Geometry: final body of the model. Coordinates: model frame, mm. A direction names the side the tool comes from. Give positions to 0.01 mm unless a question says otherwise; leave off trailing zeros. Write each loop counter-clockwise with the first axis right and the second up, starting at its lowest first coordinate (ties: lowest second). Pieces come first, ordered by that corner, then holes. Notation, with made-up numbers: (57.25, -22.5) -> (97.25, -22.5) arc R21 cw to (97.25, 16.5) -> close; hole circle Ø8 at (21.5, 42). An arc over 180 degrees is marked (long way). Use CSV: the item, a comma, the result in double quotes. Start each with the question number.
1) Set-up query: faces 1 (the face through (0, 12, 1)), 2 (the face through (0, 5, 2.5)). Return all of +Z, -Z, +X, -X, +Y, -Y with unobstructed straight access to the full face (end or side cutting, diameter ignored); none if empty.
2) Section B-B (x = 0). Output: boundary loops of the cut face in (y, z), plus the area to 3 significant figures.
3) Contact query for flat-ended pins moving along their axis: P1, Ø2, axis at y = -9.5, z = 3.5, coming from the -X side; P2, Ø1.5, axis at x = -2, z = 2.5, coming from the -Y side; P3, Ø2, axis at y = -15, z = 1.5, coming from the +X side; P4, Ø5, axis at x = 0, y = 0, coming from the +Z side. Output: stop coordinate, or through.
4) Material intervals for line 1 (X direction, y = 0, z = 0.8); line 2 (X direction, y = 0, z = 2.05); line 3 (Z direction, x = 1.5, y = 9), sorted ascending. Write a range as [from, to].
5) Section C-C (z = 0.6). Output: boundary loops of the cut face in (x, y).
6) Draft query along Y for faces 3 (the face through (1, -16, 4)), 4 (the face through (0.148, -6.157, 2.533)), 5 (the face through (-10, 0, 1)). Return one class per face: pulls with the +Y half, pulls with the -Y half, needs draft (parallel to the pull), parting line crosses it, or undercut.
7) Section D-D (y = -15). Output: boundary loops of the cut face in (x, z), plus the area to 3 significant figures.
8) Section A-A (y = 0). Output: boundary loops of the cut face in (x, z).
```python
from build123d import *

# Parameters (mm, degrees)
ESQUISSE1_R             = 4
ESQUISSE1_R_2           = 1.2
ESQUISSE1_R_3           = 1.5
BOSS_EXTRU_1_DEPTH      = 4
ENL_V_MAT_EXTRU_1_DEPTH = 25
CHANFREIN1_SIZE         = 1
CONG_1_R                = 4


with BuildPart() as part:
    # Esquisse1 → Boss.-Extru.1 (new body)
    with BuildSketch(Plane.XY):
        with BuildLine():
            Line((-10.150862032, -6.4), (-3.383620677, -17.133333333))
            ThreePointArc((-3.383620677, -17.133333333), (0, -19), (3.383620677, -17.133333333))
            Line((3.383620677, -17.133333333), (10.150862032, -6.4))
            ThreePointArc((10.150862032, -6.4), (0, 12), (-10.150862032, -6.4))
        make_face()
        Circle(ESQUISSE1_R, mode=Mode.SUBTRACT)
        with Locations((0, -15)):
            Circle(ESQUISSE1_R_2, mode=Mode.SUBTRACT)
        with Locations((-8.5, 0)):
            Circle(ESQUISSE1_R_3, mode=Mode.SUBTRACT)
        with Locations((8.5, 0)):
            Circle(ESQUISSE1_R_3, mode=Mode.SUBTRACT)
    extrude(amount=BOSS_EXTRU_1_DEPTH)

    # Esquisse2 → Enlèv. mat.-Extru.1 (cut, symmetric)
    with BuildSketch(Plane(origin=(0, 0, 0), x_dir=(0, 0, -1), z_dir=(1, 0, 0))):
        Polygon((-4, -11.766666667), (-2.5, -6.168590455), (-2.5, 12), (-4, 12), align=None)
    extrude(amount=ENL_V_MAT_EXTRU_1_DEPTH, both=True, mode=Mode.SUBTRACT)

    # Chanfrein1
    chanfrein1_edges = [part.edges().sort_by_distance(p)[0] for p in [
        (-10, 0, 2.5),
        (7, 0, 2.5),
    ]]
    chamfer(chanfrein1_edges, length=CHANFREIN1_SIZE)

    # Congé1
    cong_1_edges = [part.edges().sort_by_distance(p)[0] for p in [
        (0, -6.168590455, 2.5),
        (0, -11.766666667, 4),
    ]]
    fillet(cong_1_edges, radius=CONG_1_R)


solid = part.part
```
Answers follow:
1,face 1,"+Z, -Z"
1,face 2,"+Z, +X, -X, +Y"
2,outline,"(-19, 0) -> (-16.2, 0) -> (-16.2, 4) -> (-19, 4) -> close; (-13.8, 0) -> (-4, 0) -> (-4, 2.5) -> (-5.64, 2.5) arc R4 cw to (-6.68, 2.64) -> (-11.26, 3.86) arc R4 ccw to (-12.29, 4) -> (-13.8, 4) -> close; (4, 0) -> (12, 0) -> (12, 2.5) -> (4, 2.5) -> close"
2,area,"62.9 mm^2"
3,P1,"stops at x = -8.79"
3,P2,"stops at y = -18.8"
3,P3,"stops at x = 5.36"
3,P4,"passes through"
4,line 1,"x = [-12, -10], [-7, -4], [4, 7], [10, 12]"
4,line 2,"x = [-12, -10.55], [-6.45, -4], [4, 6.45], [10.55, 12]"
4,line 3,"z = [0, 2.5]"
5,outline,"(-10.15, -6.4) -> (-3.38, -17.13) arc R4 ccw to (3.38, -17.13) -> (10.15, -6.4) arc R12 ccw (long way) to start; hole circle Ø3 at (-8.5, 0); hole circle Ø8 at (0, 0); hole circle Ø2.4 at (0, -15); hole circle Ø3 at (8.5, 0)"
6,face 3,"needs draft"
6,face 4,"pulls with the +Y half"
6,face 5,"undercut"
7,outline,"(-4.73, 0) -> (-1.2, 0) -> (-1.2, 4) -> (-4.73, 4) -> close; (1.2, 0) -> (4.73, 0) -> (4.73, 4) -> (1.2, 4) -> close"
7,area,"28.2 mm^2"
8,outline,"(-12, 0) -> (-10, 0) -> (-10, 1.5) -> (-11, 2.5) -> (-12, 2.5) -> close; (-7, 0) -> (-4, 0) -> (-4, 2.5) -> (-6, 2.5) -> (-7, 1.5) -> close; (4, 0) -> (7, 0) -> (7, 1.5) -> (6, 2.5) -> (4, 2.5) -> close; (10, 0) -> (12, 0) -> (12, 2.5) -> (11, 2.5) -> (10, 1.5) -> close"
